```python
from build123d import *

# Parameters (mm, degrees)
BOSS_EXTRUDE1_DEPTH = 4
SKETCH2_R           = 1.75
CUT_EXTRUDE1_DEPTH  = 4
FILLET1_R           = 1


with BuildPart() as part:
    # Sketch1 → Boss-Extrude1 (new body)
    with BuildSketch(Plane.XY):
        Polygon((-27, -11), (-16, -11), (-16, 0), (16, 0), (16, -11), (27, -11), (27, -4), (20, -4), (20, 4), (-20, 4), (-20, -4), (-27, -4), align=None)
    extrude(amount=BOSS_EXTRUDE1_DEPTH)

    # Sketch2 → Cut-Extrude1 (cut)
    with BuildSketch(Plane.XY.offset(4)):
        with Locations((-23.25, -7.5)):
            Circle(SKETCH2_R)
    cut_extrude1 = extrude(amount=-CUT_EXTRUDE1_DEPTH, mode=Mode.SUBTRACT)

    # Mirror1: Cut-Extrude1 across plane
    add(cut_extrude1.mirror(Plane(origin=(0, 0, 0), x_dir=(0, 0, 1), z_dir=(1, 0, 0))), mode=Mode.SUBTRACT)

    # Fillet1
    fillet1_edges = [part.edges().sort_by_distance(p)[0] for p in [
        (-27, -4, 2),
        (-20, -4, 2),
        (-20, 4, 2),
        (20, 4, 2),
        (20, -4, 2),
        (27, -4, 2),
    ]]
    fillet(fillet1_edges, radius=FILLET1_R)


solid = part.part
```
Here's how the part is built. I have some questions about the finished solid (model axes, mm). A direction names the side the tool comes from. Coordinates: 2 decimals unless noted, no trailing zeros. Order: outer loops, then holes, each group sorted by start corner. A loop starts at its lowest first (then second) coordinate and runs counter-clockwise, first axis right, second up. Notation, with made-up numbers: M -30,51.25 L 24,51.25 A10 cw 24,68.25 Z; hole C -7.75,80.25 d2. An arc over 180 degrees is marked long. Answer as a JSON object with one key per item and string values. Group by question number.
(1) For pin 1 (2 mm diameter, centred on x = 7.5, z = 2.5, fed in from -Y); pin 2 (2 mm diameter, centred on x = -23.25, y = -7.5, fed in from +Z); pin 3 (2 mm diameter, centred on y = 0, z = 2, fed in from +X), each with a flat end and sliding along its axis, tell me the tip position at first contact or that it passes through.
(2) If we mould it in two halves opening along Y, with no side actions, what happens to faces 6 (the face through (25, -7.42, 2.03)), 7 (the face through (-27, -8, 2)), 8 (the face through (-19.715, 3.699, 2.028)), 9 (the face through (-25, -7.42, 2.03))? For each: released by +Y, released by -Y, zero draft, split by the parting line, or undercut.
(3) Suppose I cut it at D-D, the plane y = -7.5. Please give me the cut outline in (x, z), then the cut area to 3 significant figures.
(4) Suppose I cut it at A-A, the plane y = -9.75. Please give me the cut outline in (x, z).
(5) Suppose I cut it at B-B, the plane x = 23.25. Please give me the cut outline in (y, z).
(6) Suppose I cut it at C-C, the plane z = 3.3. Please give me the cut outline in (x, y).
(7) I need wall thicknesses on probe 1 along Y at (x, z) = (-23.25, 3.05); probe 2 along X at (y, z) = (-9.75, 3.45); probe 3 along Y at (x, z) = (6.5, 2.4). Which ranges of each line are inside material? Lowest first, please.
(8) Which directions (+Z, -Z, +X, -X, +Y, -Y) give clear straight access to the entire face, cutting with the end or side of a thin tool? Please do faces 1 (the face through (-23, -4, 2)), 2 (the face through (21, -11, 2)), 3 (the face through (0, 2, 0)), 4 (the face through (24, -4, 2)), 5 (the face through (-16, -6, 2)).
Values found:
{
 "1": {"pin 1": "stops at y = 0", "pin 2": "passes through", "pin 3": "stops at x = 20"},
 "2": {"face 6": "undercut", "face 7": "zero draft", "face 8": "released by +Y", "face 9": "undercut"},
 "3": {"outline": "M -27,0 L -25,0 L -25,4 L -27,4 Z; M -21.5,0 L -16,0 L -16,4 L -21.5,4 Z; M 16,0 L 21.5,0 L 21.5,4 L 16,4 Z; M 25,0 L 27,0 L 27,4 L 25,4 Z", "area": "60.0 mm^2"},
 "4": {"outline": "M -27,0 L -16,0 L -16,4 L -27,4 Z; M 16,0 L 27,0 L 27,4 L 16,4 Z"},
 "5": {"outline": "M -11,0 L -9.25,0 L -9.25,4 L -11,4 Z; M -5.75,0 L -4,0 L -4,4 L -5.75,4 Z"},
 "6": {"outline": "M -27,-11 L -16,-11 L -16,0 L 16,0 L 16,-11 L 27,-11 L 27,-5 A1 ccw 26,-4 L 21,-4 A1 cw 20,-3 L 20,3 A1 ccw 19,4 L -19,4 A1 ccw -20,3 L -20,-3 A1 cw -21,-4 L -26,-4 A1 ccw -27,-5 Z; hole C -23.25,-7.5 d3.5; hole C 23.25,-7.5 d3.5"},
 "7": {"probe 1": "y = -11 to -9.25, -5.75 to -4", "probe 2": "x = -27 to -16, 16 to 27", "probe 3": "y = 0 to 4"},
 "8": {"face 1": "+Z, -Z, -X, +Y", "face 2": "+Z, -Z, +X, -X, -Y", "face 3": "-Z, +X, -X, +Y, -Y", "face 4": "+Z, -Z, +X, +Y", "face 5": "+Z, -Z, -Y"}
}
